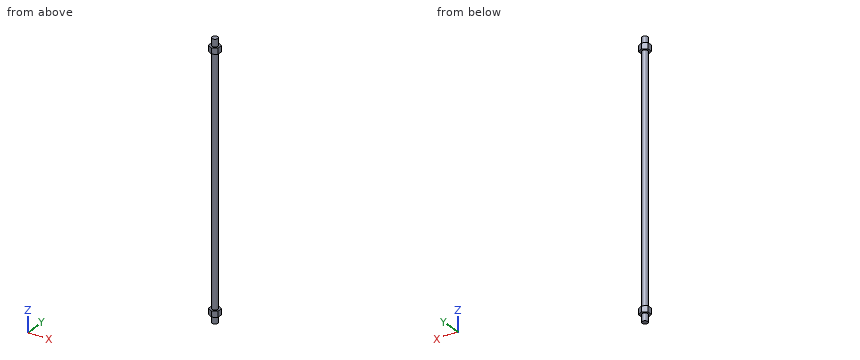
Autodesk Inventor part; units mm, degrees
ref_plane "YZ Plane" through (0, 0, 0) normal (1, 0, 0) x (0, 1, 0)
ref_plane "XZ Plane" through (0, 0, 0) normal (0, 1, 0) x (-1, 0, 0)
ref_plane "XY Plane" through (0, 0, 0) normal (0, 0, 1) x (1, 0, 0)
sketch "Эскиз1" plane through (0, 0, 0) normal (0, 0, 1) x (1, 0, 0)
  circle A0 centre (0, 0) radius 2
  dimension "d0" = 4
extrude "Выдавливание1" add sketch "Эскиз1" along normal blind 83
sketch "Эскиз2" plane through (0, 0, 83) normal (0, 0, 1) x (1, 0, 0)
  line L0 (0, 3.7538) -> (3.2509, 1.8769)
  line L1 (3.2509, 1.8769) -> (3.2509, -1.8769)
  line L2 (3.2509, -1.8769) -> (0, -3.7538)
  line L3 (0, -3.7538) -> (-3.2509, -1.8769)
  line L4 (-3.2509, -1.8769) -> (-3.2509, 1.8769)
  line L5 (-3.2509, 1.8769) -> (0, 3.7538)
  point P0 (0, 0)
  point P1 (0, 0)
extrude "Выдавливание2" add sketch "Эскиз2" along normal blind 4
sketch "Эскиз3" plane through (0, 0, 87) normal (0, 0, 1) x (1, 0, 0)
  circle A0 centre (0, 0) radius 2
  circle A1 centre (0, 0) radius 2
extrude "Выдавливание3" add sketch "Эскиз3" along normal blind 5
thread "Резьба1"
mirror "Зеркальное отражение1" about plane through (0, 0, 0) normal (0, 0, -1)
properties part number "ось пушки 2" material "Сталь, литейная"
CAD build for the part. Positions are in the model's coordinates, mm. Coordinates: 2 decimals unless noted, no trailing zeros. Loops run counter-clockwise (first coordinate to the right, second up) from the corner with the lowest first, then second, coordinate; pieces in that order, holes last. Notation, with made-up numbers: (48.5, 42.5) - (105.5, 42.5) arc R29 cw to (105.5, 81.5) - close; hole circle Ø2 at (48, 4). An arc over 180 degrees is marked (long way). Return JSON: item names as keys, results as strings.
1. Probe L1, parallel to Z at x = 0.75, y = -2.75; L2, parallel to Y at x = 0, z = 10; L3, parallel to X at y = -0.75, z = -47.5. List the from-to ranges inside material, lowest first. Write a range as from..to.
Result:
{"L1": "z = -87..-83, 83..87", "L2": "y = -2..2", "L3": "x = -1.85..1.85"}
2. Band-saw the part on B-B (z = -78). Give the cut face in (x, y), and give its area (3 significant figures).
Result:
{"outline": "circle Ø4 at (0, 0)", "area": "12.6 mm2"}
3. Drop flat-ended pins along their axis: pin 1 (4 mm diameter, centred on y = -0.5, z = -44, fed in from -X); pin 2 (1 mm diameter, centred on x = 0, z = -42.5, fed in from -Y); pin 3 (3 mm diameter, centred on y = 1, z = 20, fed in from +X). Give the stop position or say it passes through.
Result:
{"pin 1": "stops at x = -2", "pin 2": "stops at y = -2", "pin 3": "stops at x = 2"}
4. Band-saw the part on A-A (y = 0). Give the cut face in (x, z).
Result:
{"outline": "(-3.25, -87) - (-2, -87) - (-2, -92) - (2, -92) - (2, -87) - (3.25, -87) - (3.25, -83) - (2, -83) - (2, 83) - (3.25, 83) - (3.25, 87) - (2, 87) - (2, 92) - (-2, 92) - (-2, 87) - (-3.25, 87) - (-3.25, 83) - (-2, 83) - (-2, -83) - (-3.25, -83) - close"}
